For this review, take the finished solid that the model builds, in its own axes (mm). A direction names the side the tool comes from. Coordinates: 2 decimals unless noted, no trailing zeros. Loops run counter-clockwise (first coordinate to the right, second up) from the corner with the lowest first, then second, coordinate; pieces in that order, holes last. Notation, with made-up numbers: M -38,2.25 L -22,2.25 A11 ccw -22,10.25 Z; hole C 58.25,53.25 d6. An arc over 180 degrees is marked long. Write each question's results on one line, items separated by ' | '. Start each with the question number.
Autodesk Inventor part; units mm, degrees
ref_plane "YZ Plane" through (0, 0, 0) normal (1, 0, 0) x (0, 1, 0)
ref_plane "XZ Plane" through (0, 0, 0) normal (0, 1, 0) x (-1, 0, 0)
ref_plane "XY Plane" through (0, 0, 0) normal (0, 0, 1) x (1, 0, 0)
sketch "Sketch1" plane through (0, 0, 0) normal (1, 0, 0) x (0, 1, 0)
  circle A0 centre (0, 0) radius 3.175
  dimension "d0" = 6.35
extrude "Extrusion1" add sketch "Sketch1" along normal blind 25.4
thread "Thread1"
sketch "Sketch2" plane through (25.4, 0, 0) normal (1, 0, 0) x (0, 0, -1)
  circle A0 centre (0, 0) radius 6.35
  line L0 (6.35, 0) -> (3.175, -5.4993)
  line L1 (3.175, -5.4993) -> (-3.175, -5.4993)
  line L2 (-3.175, -5.4993) -> (-6.35, 0)
  line L3 (-6.35, 0) -> (-3.175, 5.4993)
  line L4 (-3.175, 5.4993) -> (3.175, 5.4993)
  line L5 (3.175, 5.4993) -> (6.35, 0)
  dimension "d5" = 12.7
extrude "Extrusion2" add sketch "Sketch2" along normal blind 3.9688 contours L0 L1 L2 L3 L4 L5
properties part number "bolt"
Q1. Take a section at C-C, the plane y = 1. Give the boundary of the cut face in (x, z).
Q2. For faces 1 (the face through (12.52, -0.69, 3.1)), 2 (the face through (27.36, 2.79, -4.74)), list the 3-axis set-ups (+Z, -Z, +X, -X, +Y, -Y) from which the entire face can be reached by the end or side of a thin tool; tool diameter is ignored.
Q3. Insertion check: P1, Ø2, axis at x = 19.5, z = -2, coming from the -Y side; P2, Ø5, axis at x = 23.5, z = 1, coming from the +Y side; P3, Ø1.5, axis at x = 11.5, z = -2, coming from the +Y side; P4, Ø1.5, axis at x = 16.5, z = -1.5, coming from the -Y side. Each pin has a flat end and moves straight along its axis. Give the tip position at first contact, or say it passes through.
Q4. Take a section at B-B, the plane x = 2.25. Give the boundary of the cut face in (y, z) (3 decimals), then the cut area to 3 significant figures.
Q5. Take a section at D-D, the plane y = 3.5. Give the boundary of the cut face in (x, z), then the cut area to 3 significant figures.
Q6. To check wall thickness, follow line 1 along X through (y, z) = (-1, -4); line 2 along Y through (x, z) = (3.5, 2.25); line 3 along Z through (x, y) = (2.5, -2.5). State the ranges of each line that lie inside material, in increasing order.
Q7. Take a section at A-A, the plane z = -0.5. Give the boundary of the cut face in (x, y), then the cut area to 3 significant figures.
Results:
1) outline: M 0,-3.01 L 25.4,-3.01 L 25.4,-5.77 L 29.37,-5.77 L 29.37,5.77 L 25.4,5.77 L 25.4,3.01 L 0,3.01 Z
2) face 1: -X | face 2: -Z, +X, -X, +Y
3) P1: y = -3.01 | P2: y = 5.5 | P3: y = 2.92 | P4: y = -3.09
4) outline: C 0,0 d6.35 | area: 31.7 mm^2
5) outline: M 25.4,-4.33 L 29.37,-4.33 L 29.37,4.33 L 25.4,4.33 Z | area: 34.4 mm^2
6) line 1: 25.4 to 29.37 | line 2: -2.24 to 2.24 | line 3: -1.96 to 1.96
7) outline: M 0,-3.14 L 25.4,-3.14 L 25.4,-5.5 L 29.37,-5.5 L 29.37,5.5 L 25.4,5.5 L 25.4,3.14 L 0,3.14 Z | area: 203 mm^2
